from build123d import *

# Parameters (mm, degrees)
F1_DEPTH  = 80
F2_R      = 5
F3_DEPTH  = 25
F5_DEPTH  = 60
F6_R      = 35
F7_DEPTH  = 33.666907
F8_R      = 25
F9_DEPTH  = 52.6
F11_DEPTH = 25


with BuildPart() as f1:
    # F0 (on Front) → F1 (new body)
    with BuildSketch(Plane.XZ):
        Polygon((120, 0), (0, 0), (0, -15), (30, -15), (30, -10), (90, -10), (90, -15), (120, -15), align=None)
    extrude(amount=F1_DEPTH)

    # F2 (on face) → F3 (cut)
    with BuildSketch(Plane.XY):
        with Locations((15, -15)):
            Circle(F2_R)
        with Locations((15, -65)):
            Circle(F2_R)
        with Locations((105, -65)):
            Circle(F2_R)
        with Locations((105, -15)):
            Circle(F2_R)
    extrude(amount=-F3_DEPTH, mode=Mode.SUBTRACT)

    # F4 (on face) → F5 (join)
    with BuildSketch(Plane.XY):
        Polygon((35, -45), (80, -45), (80, -56.833453), (90, -56.833453), (90, -45), (90, -35), (90, -23.166547), (80, -23.166547), (80, -35), (35, -35), align=None)
    extrude(amount=F5_DEPTH)

    # F6 (on face) → F7 (join, through all)
    with BuildSketch(Plane.XZ.offset(56.833453)):
        with Locations((85, 60)):
            Circle(F6_R)
    extrude(amount=-F7_DEPTH)

    # F8 (on face) → F9 (cut)
    with BuildSketch(Plane.XZ.offset(56.833453)):
        with Locations((85, 60)):
            Circle(F8_R)
    extrude(amount=-F9_DEPTH, mode=Mode.SUBTRACT)

    # F10 (on face) → F11 (cut)
    with BuildSketch(Plane.XZ.offset(45)):
        Polygon((35, 60), (35, 0), (50, 60), align=None)
    extrude(amount=-F11_DEPTH, mode=Mode.SUBTRACT)


solid = f1.part
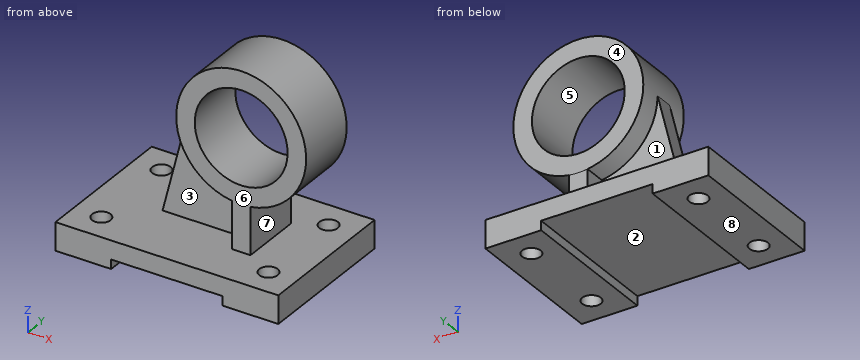
Part model, mm, in its own coordinate system. Face numbers are marked on the shaded views. A direction names the side the tool comes from. Coordinates: 2 decimals unless noted, no trailing zeros. Loops run counter-clockwise (first coordinate to the right, second up) from the corner with the lowest first, then second, coordinate; pieces in that order, holes last. Notation, with made-up numbers: (-3.75, 71.25) -> (19.25, 71.25) arc R26 ccw to (19.25, 90.25) -> close; hole circle Ø4 at (-17.5, -11.5). An arc over 180 degrees is marked (long way). Use a Markdown table: item, result. Add a question column.
Item 1: Band-saw the part on B-B on y = -15. Write the cut outline in (x, z).
Item 2: Band-saw the part on C-C on z = -5.5. Write the cut outline in (x, y).
Item 3: Band-saw the part on D-D on x = 15. Write the cut outline in (y, z).
Item 4: Flat gauge pins, fed straight in: P1, Ø20.5, axis at y = -47, z = 13, coming from the +X side; P2, Ø11.5, axis at x = 105, y = -65, coming from the +Z side; P3, Ø24, axis at x = 61.5, y = -21.5, coming from the +Z side; P4, Ø9, axis at x = 105, y = -15, coming from the +Z side. Where does each tip first touch, or does it go through?
Item 5: Probe probe 1 along Y at (x, z) = (105, -12); probe 2 along Z at (x, y) = (85, -40); probe 3 along Z at (x, y) = (73.5, -48). List the from-to ranges inside material, lowest first.
Item 6: Which spindle directions (+Z, -Z, +X, -X, +Y, -Y) get a long thin tool onto all of the face, cutting with end or side? Do the marked faces 1, 2, 3 and 4. Say none if no direction does.
Item 7: Pull direction Z, two halves, no side cores. Call the marked faces 5, 6, 7 and 8: +Z half, -Z half, draft (parallel to the pull), parting line (faces both ways), or undercut.
Geometry says:
| question | item | result |
|---|---|---|
| 1 | outline | (0, -15) -> (10, -15) -> (10, 0) -> (0, 0) -> close; (20, -15) -> (30, -15) -> (30, -10) -> (90, -10) -> (90, -15) -> (100, -15) -> (100, 0) -> (20, 0) -> close; (110, -15) -> (120, -15) -> (120, 0) -> (110, 0) -> close |
| 2 | outline | (0, -80) -> (120, -80) -> (120, 0) -> (0, 0) -> close; hole circle Ø10 at (15, -65); hole circle Ø10 at (15, -15); hole circle Ø10 at (105, -65); hole circle Ø10 at (105, -15) |
| 3 | outline | (-80, -15) -> (-70, -15) -> (-70, 0) -> (-80, 0) -> close; (-60, -15) -> (-20, -15) -> (-20, 0) -> (-60, 0) -> close; (-10, -15) -> (0, -15) -> (0, 0) -> (-10, 0) -> close |
| 4 | P1 | x = 90 |
| 4 | P2 | z = 0 |
| 4 | P3 | z = 93.02 |
| 4 | P4 | through |
| 5 | probe 1 | -80 to -70, -60 to -20, -10 to 0 |
| 5 | probe 2 | -10 to 35, 85 to 95 |
| 5 | probe 3 | -10 to 0, 26.94 to 37.8, 82.2 to 93.06 |
| 6 | face 1 | -X, +Y |
| 6 | face 2 | -Z, +Y, -Y |
| 6 | face 3 | -X, -Y |
| 6 | face 4 | +Z, +X, -X, +Y |
| 7 | face 5 | undercut |
| 7 | face 6 | draft |
| 7 | face 7 | undercut |
| 7 | face 8 | -Z half |
